The listing builds one solid part. Answer for the finished solid, in the listing's coordinates (mm). Face numbers are marked on the shaded views. A direction names the side the tool comes from. Round coordinates to 2 decimals unless told otherwise and drop trailing zeros. Order: outer loops, then holes, each group sorted by start corner. A loop starts at its lowest first (then second) coordinate and runs counter-clockwise, first axis right, second up. Notation, with made-up numbers: (13, -12.75) - (38, -12.75) arc R27 ccw to (38, 18.25) - close; hole circle Ø5 at (8, 74.25). An arc over 180 degrees is marked (long way). One line per item, written item: value. Start each with the question number.
1. Section D-D, the plane x = 10.5 is taken. Give the vertices of the cut face in (y, z).
2. Straight lines are drawn through the part: line 1 (X direction, y = 6.25, z = 8.75); line 2 (Z direction, x = 10.5, y = 3.25); line 3 (X direction, y = 1.5, z = 14.25). For each, find the intervals that lie inside material, in ascending order.
3. Section C-C, the plane y = 11.75 is taken. Give the vertices of the cut face in (x, z), then the cut area to 3 significant figures.
4. For a pull along Z with two mould halves and no side action, classify the marked faces 5, 6 and 7 as released by +Z, released by -Z, zero draft, split by the parting line, or undercut.
5. Flat-ended cylindrical pins translate along their axes: P1, Ø6.5, axis at x = 11, z = 12.5, coming from the +Y side; P2, Ø3, axis at y = 14.5, z = 10.5, coming from the +X side; P3, Ø1.6, axis at x = 10, y = 4, coming from the -Z side. Find the tip coordinate at first contact, or state that the pin passes through.
6. Section B-B, the plane z = 6 is taken. Give the vertices of the cut face in (x, y), then the cut area to 3 significant figures.
7. Section A-A, the plane y = 4.5 is taken. Give the vertices of the cut face in (x, z), then the cut area to 3 significant figures.
8. A tool of negligible diameter and unlimited length cuts with its end or side. For the marked faces 1, 2, 3 and 4, from which of +Z, -Z, +X, -X, +Y, -Y can it reach the whole face along a straight path? Write none if from no direction.
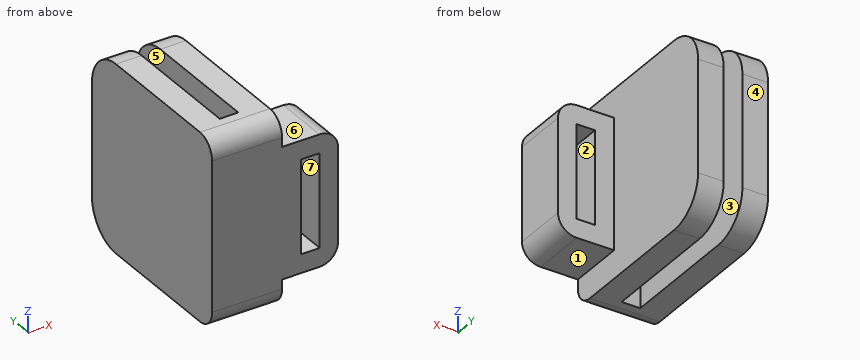
from build123d import *

# Parameters (mm, degrees)
PAD_DEPTH       = 20
SKETCH001_W     = 6
SKETCH001_H     = 14
PAD001_DEPTH    = 6
SKETCH002_W     = 2
SKETCH002_H     = 10
POCKET_DEPTH    = 10
FILLET_R        = 2
FILLET001_R     = 2
FILLET002_R     = 4
SKETCH003_W     = 2
SKETCH003_H     = 20
POCKET001_DEPTH = 17


with BuildPart() as part:
    # Sketch → Pad (new body)
    with BuildSketch(Plane.XY):
        Polygon((0, 0), (0, 20), (3, 20), (3, 3), (4.5, 3), (4.5, 20), (7.5, 20), (7.5, 0), align=None)
    extrude(amount=PAD_DEPTH)

    # Sketch001 (on Face7 of Pad) → Pad001 (join)
    with BuildSketch(Plane.YZ.offset(7.5)):
        with Locations((3, 10)):
            Rectangle(SKETCH001_W, SKETCH001_H)
    extrude(amount=PAD001_DEPTH)

    # Sketch002 (on Face7 of Pad001) → Pocket (cut)
    with BuildSketch(Plane.XZ):
        with Locations((10.531835, 10)):
            Rectangle(SKETCH002_W, SKETCH002_H)
    extrude(amount=-POCKET_DEPTH, mode=Mode.SUBTRACT)

    # Fillet
    fillet_edges = [part.edges().sort_by_distance(p)[0] for p in [
        (3.75, 0, 20),
        (3.75, 0, 0),
    ]]
    fillet(fillet_edges, radius=FILLET_R)

    # Fillet001
    fillet001_edges = [part.edges().sort_by_distance(p)[0] for p in [
        (13.5, 3, 17),
        (13.5, 3, 3),
    ]]
    fillet(fillet001_edges, radius=FILLET001_R)

    # Fillet002
    fillet002_edges = [part.edges().sort_by_distance(p)[0] for p in [
        (1.5, 20, 20),
        (6, 20, 20),
        (6, 20, 0),
        (1.5, 20, 0),
    ]]
    fillet(fillet002_edges, radius=FILLET002_R)

    # Sketch003 (on DatumPlane) → Pocket001 (cut)
    with BuildSketch(Plane(origin=(0, 20, 0), x_dir=(-1, 0, 0), z_dir=(0, 1, 0))):
        with Locations((-3.75, 10)):
            Rectangle(SKETCH003_W, SKETCH003_H)
    extrude(amount=-POCKET001_DEPTH, mode=Mode.SUBTRACT)


solid = part.part
Answer list:
1. outline: (0, 3) - (6, 3) - (6, 5) - (0, 5) - close; (0, 15) - (6, 15) - (6, 17) - (0, 17) - close
2. line 1: x = 0 to 2.75, 4.75 to 7.5
2. line 2: z = 3 to 5, 15 to 17
2. line 3: x = 0 to 9.53, 11.53 to 13.5
3. outline: (0, 0) - (2.75, 0) - (2.75, 20) - (0, 20) - close; (4.75, 0) - (7.5, 0) - (7.5, 20) - (4.75, 20) - close
3. area: 110 mm²
4. face 5: zero draft
4. face 6: released by +Z
4. face 7: undercut
5. P1: stops at y = 6
5. P2: stops at x = 7.5
5. P3: stops at z = 3
6. outline: (0, 0) - (9.53, 0) - (9.53, 6) - (7.5, 6) - (7.5, 20) - (4.75, 20) - (4.75, 3) - (2.75, 3) - (2.75, 20) - (0, 20) - close; (11.53, 0) - (13.5, 0) - (13.5, 6) - (11.53, 6) - close
6. area: 140 mm²
7. outline: (0, 0) - (2.75, 0) - (2.75, 20) - (0, 20) - close; (4.75, 0) - (7.5, 0) - (7.5, 3) - (11.5, 3) arc R2 ccw to (13.5, 5) - (13.5, 15) arc R2 ccw to (11.5, 17) - (7.5, 17) - (7.5, 20) - (4.75, 20) - close; hole (9.53, 5) - (11.53, 5) - (11.53, 15) - (9.53, 15) - close
7. area: 172 mm²
8. face 1: -Z, +X, +Y, -Y
8. face 2: +Y, -Y
8. face 3: +Z, -Z, +Y
8. face 4: +Z, -Z, +X, -X, +Y
